Here's how the part is built. I have some questions about the finished solid (model axes, mm). A direction names the side the tool comes from. Coordinates: 2 decimals unless noted, no trailing zeros. Loops run counter-clockwise (first coordinate to the right, second up) from the corner with the lowest first, then second, coordinate; pieces in that order, holes last. Notation, with made-up numbers: (-13.75, 31.5) -> (40.25, 31.5) arc R17 cw to (40.25, 53.5) -> close; hole circle Ø7 at (70, 67.5). An arc over 180 degrees is marked (long way). Answer as a JSON object with one key per item and string values. Group by question number.
Q1. I'm going to push flat-ended pins straight in: pin 1 (0.7 mm diameter, centred on y = 67, z = -9.5, fed in from -X); pin 2 (2 mm diameter, centred on x = 1, y = 79, fed in from +Z). Where does each tip first touch, or does it pass through?
Q2. On a 3-axis mill with a long thin cutter (end or side, diameter ignored), from which of +Z, -Z, +X, -X, +Y, -Y can I reach the whole of each face in a straight line? I mean faces 4 (the flat face through (6, 59, -10)), 5 (the flat face through (-4.55, 59.16, 5.54)). Say none if no direction works.
Q3. I need wall thicknesses on line 1 (Z direction, x = -9, y = 45); line 2 (Z direction, x = 0, y = 45.5); line 3 (X direction, y = 12, z = -3.5). Which ranges of each line are inside material? Lowest first, please.
Q4. Thinking about a two-plate mould opening in Z: for faces 1 (the flat face through (5, 59, 8.6)), 2 (the cylindrical face through (0, 59, -4)), 3 (the flat face through (10, 59, -6)), which applies, released by +Z, released by -Z, zero draft, split by the parting line, or undercut?
Q5. I want a section at B-B on x = 0. Write out the boundary of the cut face in (y, z).
Q6. I want a section at A-A on z = 0. Write out the boundary of the cut face in (x, y).
```python
from build123d import *

# Parameters (mm, degrees)
SKETCH1_R           = 2.5
BOSS_EXTRUDE1_DEPTH = 120
FILLET1_R           = 0.5
FILLET2_R           = 1


with BuildPart() as part:
    # Sketch1 → Boss-Extrude1 (new body)
    with BuildSketch(Plane(origin=(0, 0, 0), x_dir=(1, 0, 0), z_dir=(0, 1, 0))):
        with BuildLine():
            Line((3.2, 10), (3.2, 8.6))
            Line((3.2, 8.6), (7.610050506, 8.6))
            Line((7.610050506, 8.6), (2.289805316, 3.27975481))
            ThreePointArc((2.289805316, 3.27975481), (0, 4), (-2.289805316, 3.27975481))
            Line((-2.289805316, 3.27975481), (-7.610050506, 8.6))
            Line((-7.610050506, 8.6), (-3.2, 8.6))
            Line((-3.2, 8.6), (-3.2, 10))
            Line((-3.2, 10), (-10, 10))
            Line((-10, 10), (-10, 3.2))
            Line((-10, 3.2), (-8.6, 3.2))
            Line((-8.6, 3.2), (-8.6, 7.610050506))
            Line((-8.6, 7.610050506), (-3.27975481, 2.289805316))
            ThreePointArc((-3.27975481, 2.289805316), (-4, 0), (-3.27975481, -2.289805316))
            Line((-3.27975481, -2.289805316), (-8.6, -7.610050506))
            Line((-8.6, -7.610050506), (-8.6, -3.2))
            Line((-8.6, -3.2), (-10, -3.2))
            Line((-10, -3.2), (-10, -10))
            Line((-10, -10), (-3.2, -10))
            Line((-3.2, -10), (-3.2, -8.6))
            Line((-3.2, -8.6), (-7.610050506, -8.6))
            Line((-7.610050506, -8.6), (-2.289805316, -3.27975481))
            ThreePointArc((-2.289805316, -3.27975481), (0, -4), (2.289805316, -3.27975481))
            Line((2.289805316, -3.27975481), (7.610050506, -8.6))
            Line((7.610050506, -8.6), (3.2, -8.6))
            Line((3.2, -8.6), (3.2, -10))
            Line((3.2, -10), (10, -10))
            Line((10, -10), (10, -3.2))
            Line((10, -3.2), (8.6, -3.2))
            Line((8.6, -3.2), (8.6, -7.610050506))
            Line((8.6, -7.610050506), (3.27975481, -2.289805316))
            ThreePointArc((3.27975481, -2.289805316), (4, 0), (3.27975481, 2.289805316))
            Line((3.27975481, 2.289805316), (8.6, 7.610050506))
            Line((8.6, 7.610050506), (8.6, 3.2))
            Line((8.6, 3.2), (10, 3.2))
            Line((10, 3.2), (10, 10))
            Line((10, 10), (3.2, 10))
        make_face()
        Circle(SKETCH1_R, mode=Mode.SUBTRACT)
    extrude(amount=BOSS_EXTRUDE1_DEPTH)

    # Fillet1
    fillet1_edges = [part.edges().sort_by_distance(p)[0] for p in [
        (8.6, 60, -7.610050506),
        (8.6, 60, 7.610050506),
        (7.610050506, 60, 8.6),
        (-7.610050506, 60, 8.6),
        (-8.6, 60, 7.610050506),
        (-8.6, 60, -7.610050506),
        (-7.610050506, 60, -8.6),
        (7.610050506, 60, -8.6),
    ]]
    fillet(fillet1_edges, radius=FILLET1_R)

    # Fillet2
    fillet2_edges = [part.edges().sort_by_distance(p)[0] for p in [
        (10, 60, 10),
        (-10, 60, 10),
        (-10, 60, -10),
        (10, 60, -10),
    ]]
    fillet(fillet2_edges, radius=FILLET2_R)


solid = part.part
```
Result set:
{
 "1": {"pin 1": "stops at x = -9.99", "pin 2": "stops at z = 4"},
 "2": {"face 4": "-Z, +X, -X, +Y, -Y", "face 5": "+Y, -Y"},
 "3": {"line 1": "z = -10 to -3.2, 3.2 to 10", "line 2": "z = -4 to -2.5, 2.5 to 4", "line 3": "x = -10 to -8.6, -4.49 to -2.51, -1.94 to 1.94, 2.51 to 4.49, 8.6 to 10"},
 "4": {"face 1": "undercut", "face 2": "released by -Z", "face 3": "zero draft"},
 "5": {"outline": "(0, -4) -> (120, -4) -> (120, -2.5) -> (0, -2.5) -> close; (0, 2.5) -> (120, 2.5) -> (120, 4) -> (0, 4) -> close"},
 "6": {"outline": "(-4, 0) -> (-2.5, 0) -> (-2.5, 120) -> (-4, 120) -> close; (2.5, 0) -> (4, 0) -> (4, 120) -> (2.5, 120) -> close"}
}
